Verification items for the finished model (mm, model axes). A direction names the side the tool comes from. Give positions to 0.01 mm unless a question says otherwise; leave off trailing zeros. Order: outer loops, then holes, each group sorted by start corner. A loop starts at its lowest first (then second) coordinate and runs counter-clockwise, first axis right, second up. Notation, with made-up numbers: (-39.75, 81.5) - (16.25, 81.5) arc R8 ccw to (16.25, 94.5) - close; hole circle Ø5 at (79.25, 88). An arc over 180 degrees is marked (long way). Answer as a JSON object with one key per item and string values. Group by question number.
(1) Thickness scan on line 1 (X direction, y = -6, z = 27); line 2 (X direction, y = -9, z = 37.5); line 3 (X direction, y = -1.5, z = 33.5). Record the ranges inside material, lowest first.
(2) Access from +Z, -Z, +X, -X, +Y, -Y to the whole of each face (thin tool, end or side, straight path). Record for faces 1 (the face through (29.816, -24.564, 38.759)), 2 (the face through (18.3, -15.6, 38.3)).
(3) Section check C-C (z = -15.5). Record the boundary of the cut face in (x, y), then the cut area to 3 significant figures.
(4) Section check B-B (y = -22). Record the boundary of the cut face in (x, z).
(5) Mould release check, pull along X, two halves, no side actions. Record for faces 3 (the face through (94.205, -13, 16)), 4 (the face through (29.8, -15.3, 50.4)), 5 (the face through (19, -5.588, 30)): +X half, -X half, draft (parallel to the pull), parting line (faces both ways), or undercut.
(6) Depth check by flat-ended pin: pin 1 Ø2 at (x, y) = (18.5, -17) entering from +Z; pin 2 Ø8 at (x, y) = (16, -18.5) entering from +Z. Enter the tip coordinate at first touch or a pass-through.
(7) Section check D-D (y = -16). Record the boundary of the cut face in (x, z), then the cut area to 3 significant figures.
```python
from build123d import *

# Parameters (mm, degrees)
F0_W        = 127
F0_H        = 76.2
F0_R        = 6.35
F1_DEPTH    = 25.4
F2_R        = 8.1972505448
F3_DEPTH    = 19.812
F4_SIZE     = 12.7
F5_SIZE     = 5.08
F6_T1_DEPTH = 153.3415311919
F7_SIZE     = 5.08
F8_T1_DEPTH = 153.3972220228
F9_R        = 25.39999


# Not quite as in the source:
# - a fillet or chamfer that OpenCascade refuses, or shapes differently, is made with other operations: its cross-section is extruded or revolved along the edge and cut away or added
# - a fillet or chamfer is up to 0.001 mm smaller than in the source, because OpenCascade refuses the exact size


with BuildPart() as f1:
    # F0 (on Front) → F1 (new body)
    with BuildSketch(Plane.XZ):
        with Locations((30.7051779926, 16.4221930265)):
            Rectangle(F0_W, F0_H)
        with Locations((75.1551779926, 29.1221930265)):
            Circle(F0_R, mode=Mode.SUBTRACT)
    extrude(amount=F1_DEPTH)

    # F2 (on face) → F3 (cut)
    with BuildSketch(Plane.XZ.offset(25.4)):
        with Locations((19.3208176643, 30.1677044481)):
            Circle(F2_R)
    extrude(amount=-F3_DEPTH, mode=Mode.SUBTRACT)

    # F4
    f4_edges = [f1.edges().sort_by_distance(p)[0] for p in [
        (30.705178, -25.4, 54.522193),
    ]]
    chamfer(f4_edges, length=F4_SIZE)

    # F5
    f5_edges = [f1.edges().sort_by_distance(p)[0] for p in [
        (30.705178, -12.7, 54.522193),
    ]]
    chamfer(f5_edges, length=F5_SIZE)

    # F6: chamfer of 5.08 on 1 edges, made by hand

    # F6_s2 → F6_t1 (cut)
    with BuildSketch(Plane.YZ.offset(-45.9655876034)):
        Polygon((-21.8078975516, 45.414295475), (-25.4, 36.7421930265), (-25.4, 41.8221930265), align=None)
    extrude(amount=F6_T1_DEPTH, mode=Mode.SUBTRACT)

    # F7
    f7_edges = [f1.edges().sort_by_distance(p)[0] for p in [
        (30.705178, -21.807898, 45.414295),
    ]]
    chamfer(f7_edges, length=F7_SIZE)

    # F8: chamfer of 5.08 on 1 edges, made by hand

    # F8_s2 → F8_t1 (cut)
    with BuildSketch(Plane.YZ.offset(-45.9934330188)):
        Polygon((-19.8842048969, 47.3379881297), (-11.5987944233, 52.8741224145), (-16.2921024484, 50.9300905781), align=None)
    extrude(amount=F8_T1_DEPTH, mode=Mode.SUBTRACT)

    # F9 (radius 25.4 in the source; OpenCascade refuses exactly that, so slightly less here)
    f9_edges = [f1.edges().sort_by_distance(p)[0] for p in [
        (30.705178, -25.4, -21.677807),
    ]]
    fillet(f9_edges, radius=F9_R)


solid = f1.part
```
Solutions:
{
 "1": {"line 1": "x = -32.79 to 11.76, 26.88 to 69.17, 81.14 to 94.21", "line 2": "x = -32.79 to 15.66, 22.99 to 94.21", "line 3": "x = -32.79 to 70.56, 79.75 to 94.21"},
 "2": {"face 1": "+Z, +X, -X, -Y", "face 2": "-Y"},
 "3": {"outline": "(-32.79, -16.6) - (94.21, -16.6) - (94.21, 0) - (-32.79, 0) - close", "area": "2,110 mm2"},
 "4": {"outline": "(-32.79, -8.97) - (94.21, -8.97) - (94.21, 43.34) - (-32.79, 43.34) - close; hole circle Ø16.39 at (19.32, 30.17); hole circle Ø12.7 at (75.16, 29.12)"},
 "5": {"face 3": "+X half", "face 4": "draft", "face 5": "undercut"},
 "6": {"pin 1": "stops at z = 49.93", "pin 2": "stops at z = 50.94"},
 "7": {"outline": "(-32.79, -16) - (94.21, -16) - (94.21, 49.93) - (-32.79, 49.93) - close; hole circle Ø16.39 at (19.32, 30.17); hole circle Ø12.7 at (75.16, 29.12)", "area": "8,040 mm2"}
}
